Input: part model. Units: mm. Frame: model coordinates. A direction names the side the tool comes from. Coordinates: 2 decimals unless noted, no trailing zeros. Loops run counter-clockwise (first coordinate to the right, second up) from the corner with the lowest first, then second, coordinate; pieces in that order, holes last. Notation, with made-up numbers: (80, -31.75) - (85, -31.75) arc R19 ccw to (85, -22.75) - close; hole circle Ø8 at (44, -22). An arc over 180 degrees is marked (long way). Use one line per item in the form item = value.
from build123d import *

# Parameters (mm, degrees)
CYLINDER003_R     = 2.9
CYLINDER003_DEPTH = 1
SPHERE_ANGLE      = 180
SPHERE_ROLL_ANGLE = 90
CYLINDER002_R     = 2.5
CYLINDER002_DEPTH = 6.2


with BuildPart() as cilindro003:
    # Cylinder003 → Cylinder003 (new body)
    with BuildSketch(Plane.XY):
        Circle(CYLINDER003_R)
    extrude(amount=CYLINDER003_DEPTH)


with BuildPart() as obj1:
    # Sphere → Sphere (revolve)
    with BuildSketch(Plane.XZ):
        with BuildLine():
            ThreePointArc((0, -2.5), (2.5, 0), (0, 2.5))
            Line((0, 2.5), (0, -2.5))
        make_face()
    revolve(axis=Axis((0, 0, 0), (0, 0, 1)), revolution_arc=SPHERE_ANGLE)


with BuildPart() as obj1_1:
    # Sphere roll: moved
    add(obj1.part.rotate(Axis((0, 0, 0), (1, 0, 0)), SPHERE_ROLL_ANGLE))


with BuildPart() as obj1_2:
    # Sphere placement: moved
    add(obj1_1.part.moved(Location((0, 0, 6.2))))


with BuildPart() as funda:
    # Cylinder002 → Cylinder002 (new body)
    with BuildSketch(Plane.XY):
        Circle(CYLINDER002_R)
    extrude(amount=CYLINDER002_DEPTH)

    # Fusion001: union Cilindro003, obj1
    add(cilindro003.part)
    add(obj1_2.part)


with BuildPart() as funda_1:
    # Fusion001 placement: moved
    add(funda.part.moved(Location((0, 6, 1.5))))


solid = funda_1.part
Q1. Set-up query: faces 1 (the cylindrical face through (-2.9, 6.1, 2)), 2 (the cylindrical face through (-0.33, 8.48, 5.06)). Return all of +Z, -Z, +X, -X, +Y, -Y with unobstructed straight access to the full face (end or side cutting, diameter ignored); none if empty.
Check values:
face_1 = +Z, -Z
face_2 = +Z
Q2. Cut plane A-A, the plane x = 0. Return loops of the section in (y, z), then the cut area to 3 significant figures.
Check values:
outline = (3.1, 1.5) - (8.9, 1.5) - (8.9, 2.5) - (8.5, 2.5) - (8.5, 7.7) arc R2.5 ccw to (3.5, 7.7) - (3.5, 2.5) - (3.1, 2.5) - close
area = 41.6 mm²
Q3. First-contact query: P1, Ø2, axis at x = 0.5, z = 7, coming from the -Y side; P2, Ø2, axis at y = 8, z = 4, coming from the +X side; P3, Ø2, axis at x = -2, z = 9, coming from the +Y side. Flat tips, straight axial feed; report the tip coordinate or a pass-through.
Check values:
P1 = 3.5
P2 = 2.29
P3 = 8.08
Q4. Ray query, line 1 along Y through (x, z) = (-0.1, 6.75); line 2 along X through (y, z) = (6.05, 3.5); line 3 along Z through (x, y) = (1.05, 7.9). Return the intervals inside material, ascending. Write a range as [from, to].
Check values:
line_1 = [3.5, 8.5]
line_2 = [-2.5, 2.5]
line_3 = [1.5, 8.94]
Q5. Cut plane C-C, the plane z = 6. Return loops of the section in (x, y).
Check values:
outline = circle Ø5 at (0, 6)
Q6. Cut plane B-B, the plane y = 6. Return loops of the section in (x, z), then the cut area to 3 significant figures.
Check values:
outline = (-2.9, 1.5) - (2.9, 1.5) - (2.9, 2.5) - (2.5, 2.5) - (2.5, 7.7) arc R2.5 ccw to (-2.5, 7.7) - (-2.5, 2.5) - (-2.9, 2.5) - close
area = 41.6 mm²
Q7. Cut plane D-D, the plane z = 8. Return loops of the section in (x, y), then the cut area to 3 significant figures.
Check values:
outline = circle Ø4.96 at (0, 6)
area = 19.4 mm²
